Drawing for the job (mm, zero at the part's lowest x, y, z). Coordinates: 2 decimals unless noted, no trailing zeros. Write each loop counter-clockwise with the first axis right and the second up, starting at its lowest first coordinate (ties: lowest second). Pieces come first, ordered by that corner, then holes. Notation, with made-up numbers: (38, -36.75) -> (83, -36.75) arc R20 ccw to (83, -18.75) -> close; hole circle Ø7 at (59, 67). An arc over 180 degrees is marked (long way). Write each question's results on one line, items separated by ' | '. Start each with the question number.
Q1. Drop flat-ended pins along their axis: pin 1 Ø3 at (y, z) = (38, 39.5) entering from +X; pin 2 Ø6.5 at (x, y) = (17.5, 20) entering from -Z (1 decimal); pin 3 Ø10 at (y, z) = (13.5, 83) entering from +X; pin 4 Ø6 at (x, y) = (27, 18.5) entering from +Z. Give the stop position or say it passes through.
Q2. Drill centre lines: line 1 (Z direction, x = 8, y = 33) (1 decimal); line 2 (Y direction, x = 26, z = 25) (1 decimal); line 3 (X direction, y = 30, z = 60) (1 decimal). Where is each one in solid material? Low to high.
Q3. Saw through at B-B on x = 12. Give the cut face in (y, z), and give its area (3 significant figures).
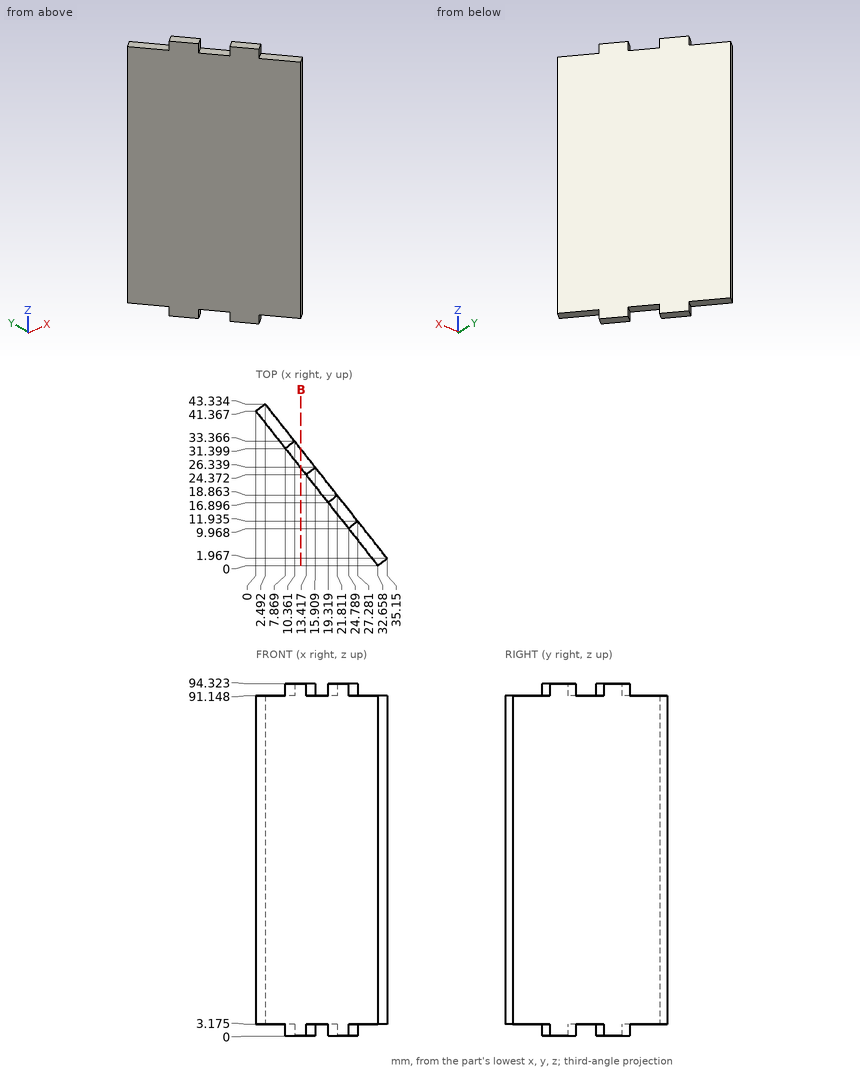
Returned:
1) pin 1: stops at x = 7.89 | pin 2: stops at z = 3.2 | pin 3: stops at x = 29.99 | pin 4: passes through
2) line 1: z = 3.2 to 91.1 | line 2: y = 8.4 to 13.6 | line 3: x = 9 to 13
3) outline: (26.17, 0) -> (31.29, 0) -> (31.29, 94.32) -> (26.17, 94.32) -> close | area: 483 mm2
